from build123d import *


with BuildPart() as part:
    # Sketch1 → Revolve1 (revolve)
    with BuildSketch(Plane.XY, mode=Mode.PRIVATE) as revolve1_sk:
        with BuildLine():
            Line((0, 0), (11.176, 0))
            Line((11.176, 0), (11.176, -15.24))
            Line((11.176, -15.24), (10.414, -15.24))
            Line((10.414, -15.24), (10.414, -21.59))
            Line((10.414, -21.59), (11.176, -21.59))
            Line((11.176, -21.59), (11.176, -41.215894229))
            Line((11.176, -41.215894229), (10.414, -41.215894229))
            Line((10.414, -41.215894229), (10.414, -47.565894229))
            Line((10.414, -47.565894229), (11.176, -47.565894229))
            Line((11.176, -47.565894229), (11.176, -67.191788457))
            add(Edge.make_bspline(
                [(11.176, -67.191788457), (11.176, -70.951410921), (10.182939744, -73.257982378), (5.810891639, -81.176539717), (5.588, -82.94585867), (5.588, -89.408)],
                knots=[0, 0, 0, 0, 0.316449847, 0.542190509, 1, 1, 1, 1], degree=3))
            Line((5.588, -89.408), (0, -89.408))
            Line((0, -89.408), (0, 0))
        make_face()
    revolve(revolve1_sk.sketch.rotate(Axis((0, -89.408, 0), (0, 1, 0)), 90), axis=Axis((0, -89.408, 0), (0, 1, 0)))


solid = part.part
Could you check a few things on this model? Use its own coordinates, in mm. A direction names the side the tool comes from. Give positions to 0.01 mm unless a question says otherwise; leave off trailing zeros. Order: outer loops, then holes, each group sorted by start corner. A loop starts at its lowest first (then second) coordinate and runs counter-clockwise, first axis right, second up. Notation, with made-up numbers: (-36.5, 25.25) -> (-13.5, 25.25) arc R20 ccw to (-13.5, 59.25) -> close; hole circle Ø5 at (-37, -1). An arc over 180 degrees is marked (long way). Answer in a Markdown table with one row per item. Add a question column.
Item 1: We'd pull the mould along Y, two halves only. Please class faces 3 (the flat face through (0, 0, 0)), 4 (the cylindrical face through (-3.128, -44.435, -9.933)), 5 (the cylindrical face through (6.8, -31.54, 8.87)): pulls with the +Y half, pulls with the -Y half, needs draft (parallel to the pull), parting line crosses it, or undercut.
Item 2: Imagine slicing it at B-B (y = -16.5). List the corners of the cut face in (x, z) for me, and give its area (3 significant figures).
Item 3: For faces 1 (the cylindrical face through (-3.128, -18.459, -9.933)), 2 (the cylindrical face through (6.8, -57.52, 8.87)), which set-ups out of +Z, -Z, +X, -X, +Y, -Y let a thin tool reach every point of the face, with its end or its side?
Item 4: I'm going to push flat-ended pins straight in: P1, Ø1, axis at x = 8, z = -6.5, coming from the -Y side; P2, Ø1, axis at x = 2, y = -21, coming from the -Z side; P3, Ø5, axis at x = 7, y = -12.5, coming from the -Z side. Where does each tip first touch, or does it pass through?
Item 5: Please list where these lines run through material, in increasing order: probe 1 along X at (y, z) = (-56, 0); probe 2 along Z at (x, y) = (0.5, -29); probe 3 along X at (y, z) = (-20, -2.25).
Item 6: Imagine slicing it at A-A (y = -31). List the corners of the cut face in (x, z) for me, and give its area (3 significant figures).
Result:
| question | item | result |
|---|---|---|
| 1 | face 3 | pulls with the +Y half |
| 1 | face 4 | undercut |
| 1 | face 5 | needs draft |
| 2 | outline | circle Ø20.83 at (0, 0) |
| 2 | area | 341 mm2 |
| 3 | face 1 | none |
| 3 | face 2 | +Y, -Y |
| 4 | P1 | y = -73.81 |
| 4 | P2 | z = -10.31 |
| 4 | P3 | z = -10.23 |
| 5 | probe 1 | -11.18 to 11.18 |
| 5 | probe 2 | -11.16 to 11.16 |
| 5 | probe 3 | -10.17 to 10.17 |
| 6 | outline | circle Ø22.35 at (0, 0) |
| 6 | area | 392 mm2 |
